from build123d import *

# Parameters (mm, degrees)
BOSS_EXTRUDE1_DEPTH  = 0.75
BOSS_EXTRUDE2_DEPTH  = 3.75
SKETCH1_4_W          = 46.25
SKETCH1_4_H          = 0.75
BOSS_EXTRUDE3_DEPTH  = 9.75
SKETCH1_5_W          = 0.75
SKETCH1_5_H          = 8
BOSS_EXTRUDE4_DEPTH  = 4.75
BOSS_EXTRUDE5_START  = 9.75
SKETCH1_8_W          = 0.75
SKETCH1_8_H          = 8
BOSS_EXTRUDE5_DEPTH  = 7
BOSS_EXTRUDE6_START  = 5.25
BOSS_EXTRUDE6_DEPTH  = 3
BOSS_EXTRUDE7_START  = 12.75
SKETCH1_11_W         = 46.25
SKETCH1_11_H         = 0.75
BOSS_EXTRUDE7_DEPTH  = 4
BOSS_EXTRUDE9_START  = 16.5
SKETCH1_12_W         = 46.25
SKETCH1_12_H         = 0.75
SKETCH1_12_W_2       = 0.75
SKETCH1_12_H_2       = 8
SKETCH1_12_H_3       = 16
BOSS_EXTRUDE9_DEPTH  = 0.75
SKETCH3_W            = 80.25
SKETCH3_H            = 3
BOSS_EXTRUDE10_DEPTH = 1.5
SKETCH6_W            = 80.25
SKETCH6_H            = 3
BOSS_EXTRUDE11_DEPTH = 1.5
SKETCH4_R            = 0.6
CUT_EXTRUDE1_DEPTH   = 79
SKETCH7_R            = 0.6
CUT_EXTRUDE2_DEPTH   = 79


with BuildPart() as part:
    # Sketch1 → Boss-Extrude1 (new body)
    with BuildSketch(Plane(origin=(0, 0, 0), x_dir=(1, 0, 0), z_dir=(0, 1, 0))):
        with BuildLine():
            Line((0.75, 51.75), (80.25, 51.75))
            ThreePointArc((80.25, 51.75), (81.310660172, 51.310660172), (81.75, 50.25))
            Line((81.75, 50.25), (81.75, 0.75))
            ThreePointArc((81.75, 0.75), (81.310660172, -0.310660172), (80.25, -0.75))
            Line((80.25, -0.75), (0.75, -0.75))
            ThreePointArc((0.75, -0.75), (-0.310660172, -0.310660172), (-0.75, 0.75))
            Line((-0.75, 0.75), (-0.75, 50.25))
            ThreePointArc((-0.75, 50.25), (-0.310660172, 51.310660172), (0.75, 51.75))
        make_face()
    extrude(amount=BOSS_EXTRUDE1_DEPTH)

    # Sketch1_3 → Boss-Extrude2 (add)
    with BuildSketch(Plane(origin=(0, 0, 0), x_dir=(1, 0, 0), z_dir=(0, 1, 0))):
        with BuildLine():
            Line((80.25, 51), (0.75, 51))
            Line((0.75, 51), (0.75, 49.5))
            Line((0.75, 49.5), (81, 49.5))
            Line((81, 49.5), (81, 50.25))
            ThreePointArc((81, 50.25), (80.780330086, 50.780330086), (80.25, 51))
        make_face()
        with BuildLine():
            Line((81, 1.5), (0.75, 1.5))
            Line((0.75, 1.5), (0.75, 0))
            Line((0.75, 0), (80.25, 0))
            ThreePointArc((80.25, 0), (80.780330086, 0.219669914), (81, 0.75))
            Line((81, 0.75), (81, 1.5))
        make_face()
    extrude(amount=BOSS_EXTRUDE2_DEPTH)

    # Sketch1_4 → Boss-Extrude3 (add)
    with BuildSketch(Plane(origin=(0, 0, 0), x_dir=(1, 0, 0), z_dir=(0, 1, 0))):
        with BuildLine():
            Line((81, 14.5), (81, 1.5))
            Line((81, 1.5), (81, 0.75))
            ThreePointArc((81, 0.75), (80.780330086, 0.219669914), (80.25, 0))
            Line((80.25, 0), (47, 0))
            Line((47, 0), (47, -0.75))
            Line((47, -0.75), (80.25, -0.75))
            ThreePointArc((80.25, -0.75), (81.310660172, -0.310660172), (81.75, 0.75))
            Line((81.75, 0.75), (81.75, 14.5))
            Line((81.75, 14.5), (81, 14.5))
        make_face()
        with BuildLine():
            Line((80.25, 51.75), (47, 51.75))
            Line((47, 51.75), (47, 51))
            Line((47, 51), (80.25, 51))
            ThreePointArc((80.25, 51), (80.780330086, 50.780330086), (81, 50.25))
            Line((81, 50.25), (81, 49.5))
            Line((81, 49.5), (81, 22.5))
            Line((81, 22.5), (81.75, 22.5))
            Line((81.75, 22.5), (81.75, 50.25))
            ThreePointArc((81.75, 50.25), (81.310660172, 51.310660172), (80.25, 51.75))
        make_face()
        with Locations((23.875, -0.375)):
            Rectangle(SKETCH1_4_W, SKETCH1_4_H)
        with Locations((23.875, 51.375)):
            Rectangle(SKETCH1_4_W, SKETCH1_4_H)
    extrude(amount=BOSS_EXTRUDE3_DEPTH)

    # Sketch1_5 → Boss-Extrude4 (add)
    with BuildSketch(Plane(origin=(0, 0, 0), x_dir=(1, 0, 0), z_dir=(0, 1, 0))):
        with Locations((81.375, 18.5)):
            Rectangle(SKETCH1_5_W, SKETCH1_5_H)
    extrude(amount=BOSS_EXTRUDE4_DEPTH)

    # Sketch1_8 → Boss-Extrude5 (add)
    with BuildSketch(Plane(origin=(0, 0, 0), x_dir=(1, 0, 0), z_dir=(0, 1, 0)).offset(BOSS_EXTRUDE5_START)):
        with BuildLine():
            Line((81, 14.5), (81, 1.5))
            Line((81, 1.5), (81, 0.75))
            ThreePointArc((81, 0.75), (80.780330086, 0.219669914), (80.25, 0))
            Line((80.25, 0), (47, 0))
            Line((47, 0), (47, -0.75))
            Line((47, -0.75), (80.25, -0.75))
            ThreePointArc((80.25, -0.75), (81.310660172, -0.310660172), (81.75, 0.75))
            Line((81.75, 0.75), (81.75, 14.5))
            Line((81.75, 14.5), (81, 14.5))
        make_face()
        with Locations((81.375, 18.5)):
            Rectangle(SKETCH1_8_W, SKETCH1_8_H)
        with BuildLine():
            Line((80.25, 51.75), (47, 51.75))
            Line((47, 51.75), (47, 51))
            Line((47, 51), (80.25, 51))
            ThreePointArc((80.25, 51), (80.780330086, 50.780330086), (81, 50.25))
            Line((81, 50.25), (81, 49.5))
            Line((81, 49.5), (81, 22.5))
            Line((81, 22.5), (81.75, 22.5))
            Line((81.75, 22.5), (81.75, 50.25))
            ThreePointArc((81.75, 50.25), (81.310660172, 51.310660172), (80.25, 51.75))
        make_face()
    extrude(amount=BOSS_EXTRUDE5_DEPTH)

    # Sketch1_9 → Boss-Extrude6 (add)
    with BuildSketch(Plane(origin=(0, 0, 0), x_dir=(1, 0, 0), z_dir=(0, 1, 0)).offset(BOSS_EXTRUDE6_START)):
        with BuildLine():
            Line((47, 51), (0.75, 51))
            Line((0.75, 51), (0.75, 49.5))
            Line((0.75, 49.5), (81, 49.5))
            Line((81, 49.5), (81, 50.25))
            ThreePointArc((81, 50.25), (80.780330086, 50.780330086), (80.25, 51))
            Line((80.25, 51), (47, 51))
        make_face()
        with BuildLine():
            Line((81, 1.5), (0.75, 1.5))
            Line((0.75, 1.5), (0.75, 0))
            Line((0.75, 0), (47, 0))
            Line((47, 0), (80.25, 0))
            ThreePointArc((80.25, 0), (80.780330086, 0.219669914), (81, 0.75))
            Line((81, 0.75), (81, 1.5))
        make_face()
    extrude(amount=BOSS_EXTRUDE6_DEPTH)

    # Sketch1_11 → Boss-Extrude7 (add)
    with BuildSketch(Plane(origin=(0, 0, 0), x_dir=(1, 0, 0), z_dir=(0, 1, 0)).offset(BOSS_EXTRUDE7_START)):
        with Locations((23.875, -0.375)):
            Rectangle(SKETCH1_11_W, SKETCH1_11_H)
        with Locations((23.875, 51.375)):
            Rectangle(SKETCH1_11_W, SKETCH1_11_H)
    extrude(amount=BOSS_EXTRUDE7_DEPTH)

    # Sketch1_12 → Boss-Extrude9 (add)
    with BuildSketch(Plane(origin=(0, 0, 0), x_dir=(1, 0, 0), z_dir=(0, 1, 0)).offset(BOSS_EXTRUDE9_START)):
        Polygon((81, 49.5), (0.75, 49.5), (0.75, 1.5), (81, 1.5), (81, 14.5), (81, 22.5), align=None)
        with BuildLine():
            Line((47, 51), (0.75, 51))
            Line((0.75, 51), (0.75, 49.5))
            Line((0.75, 49.5), (81, 49.5))
            Line((81, 49.5), (81, 50.25))
            ThreePointArc((81, 50.25), (80.780330086, 50.780330086), (80.25, 51))
            Line((80.25, 51), (47, 51))
        make_face()
        with Locations((23.875, 51.375)):
            Rectangle(SKETCH1_12_W, SKETCH1_12_H)
        with BuildLine():
            Line((81, 1.5), (0.75, 1.5))
            Line((0.75, 1.5), (0.75, 0))
            Line((0.75, 0), (47, 0))
            Line((47, 0), (80.25, 0))
            ThreePointArc((80.25, 0), (80.780330086, 0.219669914), (81, 0.75))
            Line((81, 0.75), (81, 1.5))
        make_face()
        with Locations((23.875, -0.375)):
            Rectangle(SKETCH1_12_W, SKETCH1_12_H)
        with BuildLine():
            Line((81, 14.5), (81, 1.5))
            Line((81, 1.5), (81, 0.75))
            ThreePointArc((81, 0.75), (80.780330086, 0.219669914), (80.25, 0))
            Line((80.25, 0), (47, 0))
            Line((47, 0), (47, -0.75))
            Line((47, -0.75), (80.25, -0.75))
            ThreePointArc((80.25, -0.75), (81.310660172, -0.310660172), (81.75, 0.75))
            Line((81.75, 0.75), (81.75, 14.5))
            Line((81.75, 14.5), (81, 14.5))
        make_face()
        with Locations((81.375, 18.5)):
            Rectangle(SKETCH1_12_W_2, SKETCH1_12_H_2)
        with BuildLine():
            Line((0.75, 51), (0.75, 51.75))
            ThreePointArc((0.75, 51.75), (-0.310660172, 51.310660172), (-0.75, 50.25))
            Line((-0.75, 50.25), (-0.75, 37.5))
            Line((-0.75, 37.5), (0, 37.5))
            Line((0, 37.5), (0, 49.5))
            Line((0, 49.5), (0, 50.25))
            ThreePointArc((0, 50.25), (0.219669914, 50.780330086), (0.75, 51))
        make_face()
        with BuildLine():
            Line((0.75, 49.5), (0.75, 51))
            ThreePointArc((0.75, 51), (0.219669914, 50.780330086), (0, 50.25))
            Line((0, 50.25), (0, 49.5))
            Line((0, 49.5), (0.75, 49.5))
        make_face()
        Polygon((0.75, 1.5), (0.75, 49.5), (0, 49.5), (0, 37.5), (0, 21.5), (0, 1.5), align=None)
        with Locations((-0.375, 29.5)):
            Rectangle(SKETCH1_12_W_2, SKETCH1_12_H_3)
        with BuildLine():
            Line((0, 21.5), (-0.75, 21.5))
            Line((-0.75, 21.5), (-0.75, 0.75))
            ThreePointArc((-0.75, 0.75), (-0.310660172, -0.310660172), (0.75, -0.75))
            Line((0.75, -0.75), (0.75, 0))
            ThreePointArc((0.75, 0), (0.219669914, 0.219669914), (0, 0.75))
            Line((0, 0.75), (0, 1.5))
            Line((0, 1.5), (0, 21.5))
        make_face()
        with BuildLine():
            Line((0.75, 0), (0.75, 1.5))
            Line((0.75, 1.5), (0, 1.5))
            Line((0, 1.5), (0, 0.75))
            ThreePointArc((0, 0.75), (0.219669914, 0.219669914), (0.75, 0))
        make_face()
        with BuildLine():
            Line((80.25, 51.75), (47, 51.75))
            Line((47, 51.75), (47, 51))
            Line((47, 51), (80.25, 51))
            ThreePointArc((80.25, 51), (80.780330086, 50.780330086), (81, 50.25))
            Line((81, 50.25), (81, 49.5))
            Line((81, 49.5), (81, 22.5))
            Line((81, 22.5), (81.75, 22.5))
            Line((81.75, 22.5), (81.75, 50.25))
            ThreePointArc((81.75, 50.25), (81.310660172, 51.310660172), (80.25, 51.75))
        make_face()
    extrude(amount=BOSS_EXTRUDE9_DEPTH)

    # Sketch3 → Boss-Extrude10 (add)
    with BuildSketch(Plane.XY.offset(-49.5)):
        with Locations((40.875, 6.75)):
            Rectangle(SKETCH3_W, SKETCH3_H)
    extrude(amount=BOSS_EXTRUDE10_DEPTH)

    # Sketch6 → Boss-Extrude11 (add)
    with BuildSketch(Plane(origin=(0, 0, -1.5), x_dir=(-1, 0, 0), z_dir=(0, 0, -1))):
        with Locations((-40.875, 6.75)):
            Rectangle(SKETCH6_W, SKETCH6_H)
    extrude(amount=BOSS_EXTRUDE11_DEPTH)

    # Sketch4 → Cut-Extrude1 (cut)
    with BuildSketch(Plane.ZY.offset(-0.75)):
        with Locations((-49.5, 6.75)):
            Circle(SKETCH4_R)
    extrude(amount=-CUT_EXTRUDE1_DEPTH, mode=Mode.SUBTRACT)

    # Sketch7 → Cut-Extrude2 (cut)
    with BuildSketch(Plane.ZY.offset(-0.75)):
        with Locations((-1.5, 6.75)):
            Circle(SKETCH7_R)
    extrude(amount=-CUT_EXTRUDE2_DEPTH, mode=Mode.SUBTRACT)


solid = part.part
The model under review builds one solid part; all positions refer to its coordinate system, in mm. A direction names the side the tool comes from. Round coordinates to 2 decimals unless told otherwise and drop trailing zeros. Loops run counter-clockwise (first coordinate to the right, second up) from the corner with the lowest first, then second, coordinate; pieces in that order, holes last. Notation, with made-up numbers: (37, 17) -> (54, 17) arc R12 ccw to (54, 30) -> close; hole circle Ø1 at (-35, 5). An arc over 180 degrees is marked (long way). Answer as CSV lines item,"result".
1) Draft analysis for pull direction Y (two halves, no side actions). For faces 1 (the face through (40, 0, -26)), 2 (the face through (-0.3, 0.37, 0.32)), 3 (the face through (40, 16.5, -26)), state which applies: pulls with the +Y half, pulls with the -Y half, needs draft (parallel to the pull), parting line crosses it, or undercut.
Geometry results:
face 1,"pulls with the -Y half"
face 2,"needs draft"
face 3,"undercut"
2) Add section B-B on z = -17. Write out the cut boundary in (x, y), plus the area to 3 significant figures.
Geometry results:
outline,"(-0.75, 0) -> (81.75, 0) -> (81.75, 4.75) -> (81, 4.75) -> (81, 0.75) -> (-0.75, 0.75) -> close; (-0.75, 16.5) -> (81, 16.5) -> (81, 9.75) -> (81.75, 9.75) -> (81.75, 17.25) -> (-0.75, 17.25) -> close"
area,"132 mm²"
3) Add section D-D on y = 11. Write out the cut boundary in (x, z).
Geometry results:
outline,"(47, -51.75) -> (80.25, -51.75) arc R1.5 ccw to (81.75, -50.25) -> (81.75, -0.75) arc R1.5 ccw to (80.25, 0.75) -> (47, 0.75) -> (47, 0) -> (80.25, 0) arc R0.75 cw to (81, -0.75) -> (81, -50.25) arc R0.75 cw to (80.25, -51) -> (47, -51) -> close"
4) Add section A-A on x = 43. State how many separate pieces and enclosed holes the cut face has, plus the area to 3 significant figures.
Geometry results:
separate pieces,"2"
enclosed holes,"2"
area,"123 mm²"
5) Tool access review of faces 4 (the face through (0.75, 6, -1)), 5 (the face through (40, 8.25, -50)), 6 (the face through (-0.3, 16.87, -51.32)): name each direction out of +Z, -Z, +X, -X, +Y, -Y from which nothing blocks a thin tool from reaching the whole face with its end or side.
Geometry results:
face 4,"+Z, -Z, -X"
face 5,"-X"
face 6,"-Z, -X, +Y, -Y"
6) Add section C-C on x = 63.5. Write out the cut boundary in (y, z).
Geometry results:
outline,"(0, -51.75) -> (17.25, -51.75) -> (17.25, 0.75) -> (0, 0.75) -> close; hole (0.75, -49.5) -> (3.75, -49.5) -> (3.75, -51) -> (5.25, -51) -> (5.25, -48) -> (8.25, -48) -> (8.25, -51) -> (16.5, -51) -> (16.5, 0) -> (8.25, 0) -> (8.25, -3) -> (5.25, -3) -> (5.25, 0) -> (3.75, 0) -> (3.75, -1.5) -> (0.75, -1.5) -> close; hole circle Ø1.2 at (6.75, -49.5); hole circle Ø1.2 at (6.75, -1.5)"
7) To check wall thickness, follow line 1 along Y through (x, z) = (49.5, -38.5); line 2 along Z through (x, y) = (9, 15); line 3 along Y through (x, z) = (26, -1). State the ranges of each line that lie inside material, in increasing order. Write a range as from..to.
Geometry results:
line 1,"y = 0..0.75, 16.5..17.25"
line 2,"z = -51.75..-51, 0..0.75"
line 3,"y = 0..3.75, 5.25..6.42, 7.08..8.25, 16.5..17.25"
8) For P1, Ø0.6, axis at y = 10.5, z = -51.5, coming from the -X side; P2, Ø4, axis at y = 3.5, z = -49.5, coming from the -X side; P3, Ø2, axis at y = 5.5, z = -41, coming from the -X side, all flat-tipped, find the tip position at first contact; note any pin that passes through.
Geometry results:
P1,"stops at x = 47"
P2,"stops at x = 0.75"
P3,"stops at x = 81"
